Autodesk Fusion 360 part; units mm, degrees
sketch "Skizze1" plane through (0, 0, 0) normal (0, 0, 1) x (1, 0, 0)
  line L0 (-14, 14) -> (14, 14)
  line L1 (14, 14) -> (14, -14)
  line L2 (14, -14) -> (-14, -14)
  line L3 (-14, -14) -> (-14, 14)
  arc A0 (-14, -14) -> (14, -14) centre (0, 4.2566) ccw
  line L4 (-14, 3) -> (-20.1, 3)
  line L5 (-20.1, 3) -> (-20.1, -3)
  line L6 (-20.1, -3) -> (-14, -3)
  line L7 (-14, -3) -> (-14, 3)
  circle A1 centre (-17, 0) radius 1.6
  circle A2 centre (17, 0) radius 1.6
  line L8 (14, -3) -> (20.1, -3)
  line L9 (20.1, 3) -> (14, 3)
  line L10 (14, 3) -> (14, -3)
  line L11 (20.1, -3) -> (20.1, 3)
  line L12 (0, 1.75) -> (0, 22.5)
  circle A3 centre (0, 0) radius 2
  point P0 (0, -18.75)
  dimension "d16" = 40.2
  dimension "d17" = 28
  dimension "d18" = 6.1
  dimension "d21" = 4
extrude "Extrusion1" add sketch "Skizze1" along normal blind 10 contours A3 makes body 1
extrude "Extrusion2" add sketch "Skizze1" against normal blind 9.5 separate body contours L0 L1 L2 L3 L7 L10 makes body 2
extrude "Extrusion3" add sketch "Skizze1" against normal blind 9.5 contours L2 A0 bodies 2
extrude "Extrusion4" add sketch "Skizze1" against normal blind 9.5 contours A3 bodies 1 2
extrude "Extrusion5" add sketch "Skizze1" against normal blind 3.2 contours L1 L8 L9 L10 L11 bodies 1
extrude "Extrusion6" add sketch "Skizze1" against normal blind 3.2 contours L3 L4 L5 L6 L7 bodies 1
chamfer "Fase1" distance 2 angle 45 1 edges at (14, 14, -4.75) on bodies 1
chamfer "Fase2" distance 2 angle 45 1 edges at (-14, 14, -4.75) on bodies 1
fillet "Abrundung1" radius 2 1 edges at (-14, 3, -1.6) on bodies 1
fillet "Abrundung2" radius 2 1 edges at (14, 3, -1.6) on bodies 1
fillet "Abrundung3" radius 2 1 edges at (14, -3, -1.6) on bodies 1
fillet "Abrundung4" radius 2 1 edges at (-14, -3, -1.6) on bodies 1
fillet "Abrundung5" radius 2 1 edges at (20.1, 3, -1.6) on bodies 1
fillet "Abrundung6" radius 2 1 edges at (20.1, -3, -1.6) on bodies 1
fillet "Abrundung7" radius 2 1 edges at (-20.1, 3, -1.6) on bodies 1
fillet "Abrundung8" radius 2 1 edges at (-20.1, -3, -1.6) on bodies 1
Could you check a few things on this model? Use its own coordinates, in mm. A direction names the side the tool comes from. Give positions to 0.01 mm unless a question says otherwise; leave off trailing zeros. Order: outer loops, then holes, each group sorted by start corner. A loop starts at its lowest first (then second) coordinate and runs counter-clockwise, first axis right, second up. Notation, with made-up numbers: (39.25, -37.75) - (98.25, -37.75) arc R10 ccw to (98.25, -26.75) - close; hole circle Ø9 at (18.5, 18.25). An arc over 180 degrees is marked (long way). One line per item, written item: value. Start each with the question number.
1. If I drill on probe 1 along Y at (x, z) = (-17, -2.5); probe 2 along Z at (x, y) = (-9, -4); probe 3 along X at (y, z) = (8, -4.75), over which ranges is the centre line in solid material (lowest first)?
2. Imagine slicing it at D-D on y = -7. List the corners of the cut face in (x, z) for me.
3. Imagine slicing it at A-A on x = -17. List the corners of the cut face in (y, z) for me.
4. Thinking about a two-plate mould opening in Y: for faces 4 (the face through (17, -3, -2)), 5 (the face through (15.4, 0.07, -1.58)), 6 (the face through (15.7, 1.2, -3.2)), 7 (the face through (0, 14, -5)), which applies, +Y half, -Y half, draft (parallel to the pull), parting line (faces both ways), or undercut?
5. Imagine slicing it at B-B on z = -5.5. List the corners of the cut face in (x, y) for me.
6. For faces 1 (the face through (0, 2, 5)), 2 (the face through (20.1, 0, -2)), 3 (the face through (-17, 3, -2)), which set-ups out of +Z, -Z, +X, -X, +Y, -Y let a thin tool reach every point of the face, with its end or its side?
7. Imagine slicing it at C-C on x = 0. List the corners of the cut face in (y, z) for me, plus the area to 3 significant figures.
8. For P1, Ø3, axis at x = -16, y = 0.5, coming from the -Z side; P2, Ø5, axis at y = 1.5, z = -6, coming from the -X side; P3, Ø2.5, axis at x = -17.5, z = -1, coming from the -Y side; P4, Ø12, axis at x = -1.5, y = 6, coming from the +Z side, each with a flat end and sliding along its axis, tell me the tip position at first contact or that it passes through.
Values:
1. probe 1: -3 to -1.6, 1.6 to 3
1. probe 2: -9.5 to 0
1. probe 3: -14 to 14
2. outline: (-14, -9.5) - (14, -9.5) - (14, 0) - (-14, 0) - close
3. outline: (-3, -3.2) - (-1.6, -3.2) - (-1.6, 0) - (-3, 0) - close; (1.6, -3.2) - (3, -3.2) - (3, 0) - (1.6, 0) - close
4. face 4: -Y half
4. face 5: undercut
4. face 6: draft
4. face 7: +Y half
5. outline: (-14, -14) arc R23.01 ccw to (14, -14) - (14, 12) - (12, 14) - (-12, 14) - (-14, 12) - close
6. face 1: +Z
6. face 2: +Z, -Z, +X, +Y, -Y
6. face 3: +Z, -Z, -X, +Y
7. outline: (-18.75, -9.5) - (14, -9.5) - (14, 0) - (2, 0) - (2, 10) - (-2, 10) - (-2, 0) - (-18.75, 0) - close
7. area: 351 mm²
8. P1: z = -3.2
8. P2: x = -14
8. P3: y = -3
8. P4: z = 10
